For this review, take the finished solid that the model builds, in its own axes (mm). Face numbers are marked on the shaded views. Round coordinates to 2 decimals unless told otherwise and drop trailing zeros. Write each loop counter-clockwise with the first axis right and the second up, starting at its lowest first coordinate (ties: lowest second). Pieces come first, ordered by that corner, then holes. Notation, with made-up numbers: (39, 13) - (92, 13) arc R20 ccw to (92, 47) - close; hole circle Ø2 at (56, 77.25). An arc over 180 degrees is marked (long way). One line per item, written item: value. Start each with the question number.
Q1. Add section B-B on y = 1.25. Write out the cut boundary in (x, z).
Q2. Clearance check with flat-ended pins moving along their axes: pin 1 Ø6 at (x, z) = (-2.5, 5) entering from +Y; pin 2 Ø5 at (x, y) = (10.5, 5) entering from -Z; pin 3 Ø2 at (y, z) = (-4.5, -1.5) entering from -X; pin 4 Ø3 at (y, z) = (1, 2.5) entering from +X. State where each tip first meets the part, or that it passes through.
Q3. Mouldability with a two-part tool opening along Z and no side actions: class the marked faces 1, 2, 3 and 4 as +Z half, -Z half, draft (parallel to the pull), parting line (faces both ways), or undercut.
Q4. Add section A-A on x = 0. Write out the cut boundary in (y, z).
Q5. For probe 1 along Z at (x, y) = (0, 4.25); probe 2 along Z at (x, y) = (2, -4.25); probe 3 along X at (y, z) = (0.75, -0.75), list the stretches that pass through material, from the lowest coordinate up.
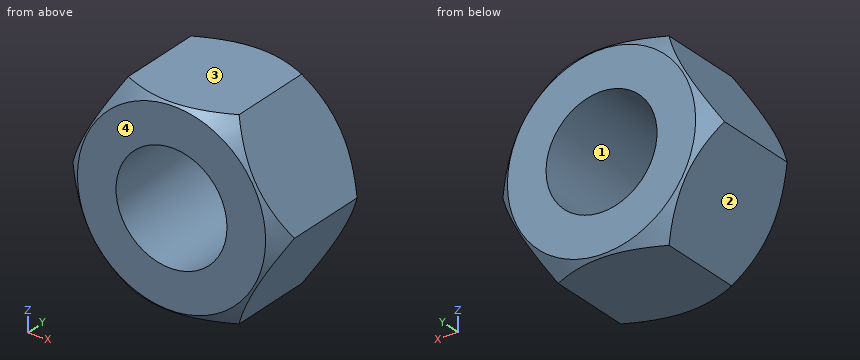
```python
from build123d import *

# Parameters (mm, degrees)
CROQUIS1_R              = 6.65
SALIENTE_EXTRUIR1_DEPTH = 7.15


with BuildPart() as part:
    # Croquis1 → Saliente-Extruir1 (new body, symmetric)
    with BuildSketch(Plane(origin=(0, 0, 0), x_dir=(1, 0, 0), z_dir=(0, 1, 0))):
        Polygon((13.279056191, 0), (6.639528096, 11.5), (-6.639528096, 11.5), (-13.279056191, 0), (-6.639528096, -11.5), (6.639528096, -11.5), align=None)
        Circle(CROQUIS1_R, mode=Mode.SUBTRACT)
    extrude(amount=SALIENTE_EXTRUIR1_DEPTH, both=True)

    # Croquis2 → Cortar-Revolución1 (revolve, cut)
    with BuildSketch(Plane.XY):
        Polygon((-11.279056191, 7.15), (-13.279056191, 5.15), (-13.279056191, 7.15), align=None)
    cortar_revoluci_n1 = revolve(axis=Axis((0, 7.15, 0), (0, 1, 0)), mode=Mode.SUBTRACT)

    # Simetría1: Cortar-Revolución1 across plane
    add(cortar_revoluci_n1.mirror(Plane.ZX), mode=Mode.SUBTRACT)


solid = part.part
```
Result set:
1. outline: (-13.28, 0) - (-6.64, -11.5) - (6.64, -11.5) - (13.28, 0) - (6.64, 11.5) - (-6.64, 11.5) - close; hole circle Ø13.3 at (0, 0)
2. pin 1: stops at y = 7.15
2. pin 2: stops at z = -9.14
2. pin 3: stops at x = -12.99
2. pin 4: stops at x = 12.7
3. face 1: undercut
3. face 2: -Z half
3. face 3: +Z half
3. face 4: draft
4. outline: (-7.15, -11.28) - (-6.93, -11.5) - (6.93, -11.5) - (7.15, -11.28) - (7.15, -6.65) - (-7.15, -6.65) - close; (-7.15, 6.65) - (7.15, 6.65) - (7.15, 11.28) - (6.93, 11.5) - (-6.93, 11.5) - (-7.15, 11.28) - close
5. probe 1: z = -11.5 to -6.65, 6.65 to 11.5
5. probe 2: z = -11.5 to -6.34, 6.34 to 11.5
5. probe 3: x = -12.85 to -6.61, 6.61 to 12.85
